from build123d import *

# Parameters (mm, degrees)
F0_W     = 136.2489163876
F0_H     = 117.116086185
F1_DEPTH = 54.356
F2_W     = 128.7117451429
F2_H     = 108.5429564118
F3_DEPTH = 54.357
F4_R     = 12.8732628807
F5_DEPTH = 136.2499163876
F6_W     = 75.9515240788
F6_H     = 23.9174129305
F7_DEPTH = 117.117086185


with BuildPart() as f1:
    # F0 (on Top) → F1 (new body)
    with BuildSketch(Plane.XY):
        Rectangle(F0_W, F0_H)
    extrude(amount=F1_DEPTH)

    # F2 (on face) → F3 (cut, through all)
    with BuildSketch(Plane.XY.offset(54.356)):
        Rectangle(F2_W, F2_H)
    extrude(amount=-F3_DEPTH, mode=Mode.SUBTRACT)

    # F4 (on face) → F5 (cut, through all)
    with BuildSketch(Plane.YZ.offset(68.1244581938)):
        with Locations((0, 37.9757620394)):
            Circle(F4_R)
    extrude(amount=-F5_DEPTH, mode=Mode.SUBTRACT)

    # F6 (on face) → F7 (cut, through all)
    with BuildSketch(Plane.XZ.offset(58.5580430925)):
        with Locations((0.5797818303, 42.3972935348)):
            Rectangle(F6_W, F6_H)
    extrude(amount=-F7_DEPTH, mode=Mode.SUBTRACT)


solid = f1.part
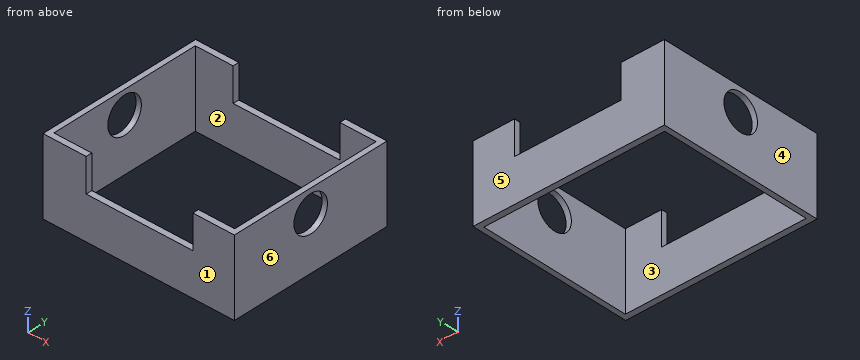
Build history of the part. All positions in model axes, mm. Face numbers are marked on the shaded views. A direction names the side the tool comes from. Give positions to 0.01 mm unless a question says otherwise; leave off trailing zeros. Order: outer loops, then holes, each group sorted by start corner. A loop starts at its lowest first (then second) coordinate and runs counter-clockwise, first axis right, second up. Notation, with made-up numbers: M 16.25,67.25 L 37.25,67.25 A25 ccw 37.25,81.25 Z; hole C -37,-26.75 d9. An arc over 180 degrees is marked long. Use one line per item in the form item = value.
Q1. Pin check, flat tip, straight feed: P1, Ø3.5, axis at x = 10.5, y = -57, coming from the +Z side. Stop position of the tip, or through.
Conclusion:
P1 = 30.44
Q2. Slice it at B-B, the plane y = 0. Write the cut outline in (x, z), and give its area (3 significant figures).
Conclusion:
outline = M -68.12,0 L -64.36,0 L -64.36,25.1 L -68.12,25.1 Z; M -68.12,50.85 L -64.36,50.85 L -64.36,54.36 L -68.12,54.36 Z; M 64.36,0 L 68.12,0 L 68.12,25.1 L 64.36,25.1 Z; M 64.36,50.85 L 68.12,50.85 L 68.12,54.36 L 64.36,54.36 Z
area = 216 mm2
Q3. Which spindle directions (+Z, -Z, +X, -X, +Y, -Y) get a long thin tool onto all of the face, cutting with end or side? Do the marked faces 1 and 2. Say none if no direction does.
Conclusion:
face_1 = +Z, -Z, +X, -X, -Y
face_2 = +Z, -Z
Q4. Pull direction X, two halves, no side cores. Call the marked faces 3, 4, 5 and 6: released by +X, released by -X, zero draft, split by the parting line, or undercut.
Conclusion:
face_3 = undercut
face_4 = released by -X
face_5 = zero draft
face_6 = released by +X
Q5. Slice it at D-D, the plane z = 41. Write the cut outline in (x, y).
Conclusion:
outline = M -68.12,-58.56 L -37.4,-58.56 L -37.4,-54.27 L -64.36,-54.27 L -64.36,-12.51 L -68.12,-12.51 Z; M -68.12,12.51 L -64.36,12.51 L -64.36,54.27 L -37.4,54.27 L -37.4,58.56 L -68.12,58.56 Z; M 38.56,-58.56 L 68.12,-58.56 L 68.12,-12.51 L 64.36,-12.51 L 64.36,-54.27 L 38.56,-54.27 Z; M 38.56,54.27 L 64.36,54.27 L 64.36,12.51 L 68.12,12.51 L 68.12,58.56 L 38.56,58.56 Z
Q6. Wall check: probe 1 along Y at (x, z) = (46, 18.5); probe 2 along X at (y, z) = (25.5, 40.5); probe 3 along Z at (x, y) = (66, 0). Give the ranges that are in metal, low to high.
Conclusion:
probe_1 = -58.56 to -54.27, 54.27 to 58.56
probe_2 = -68.12 to -64.36, 64.36 to 68.12
probe_3 = 0 to 25.1, 50.85 to 54.36
Q7. Slice it at A-A, the plane x = 0.5. Write the cut outline in (y, z), and give its area (3 significant figures).
Conclusion:
outline = M -58.56,0 L -54.27,0 L -54.27,30.44 L -58.56,30.44 Z; M 54.27,0 L 58.56,0 L 58.56,30.44 L 54.27,30.44 Z
area = 261 mm2
Q8. Slice it at C-C, the plane z = 6. Write the cut outline in (x, y), and give its area (3 significant figures).
Conclusion:
outline = M -68.12,-58.56 L 68.12,-58.56 L 68.12,58.56 L -68.12,58.56 Z; hole M -64.36,-54.27 L 64.36,-54.27 L 64.36,54.27 L -64.36,54.27 Z
area = 1,990 mm2
